Autodesk Inventor part; units mm, degrees
ref_plane "YZ Plane" through (0, 0, 0) normal (1, 0, 0) x (0, 1, 0)
ref_plane "XZ Plane" through (0, 0, 0) normal (0, 1, 0) x (-1, 0, 0)
ref_plane "XY Plane" through (0, 0, 0) normal (0, 0, 1) x (1, 0, 0)
sketch "Sketch1" plane through (0, 0, 0) normal (0, 0, 1) x (1, 0, 0)
  circle A0 centre (0, 0) radius 2.5
  dimension "d0" = 5
extrude "Extrusion1" add sketch "Sketch1" against normal blind 300
sketch "Sketch2" plane through (0, 0, 0) normal (0, 1, 0) x (-1, 0, 0)
  line L0 (1.5, -50) -> (8.5, -50)
  line L1 (8.5, -50) -> (8.5, -100)
  line L2 (8.5, -100) -> (1.5, -100)
  line L3 (1.5, -100) -> (1.5, -50)
  line L4 (1.5, -250) -> (8.5, -250)
  line L5 (8.5, -250) -> (8.5, -200)
  line L6 (8.5, -200) -> (1.5, -200)
  line L7 (1.5, -200) -> (1.5, -250)
  point P0 (0, 0)
  dimension "d3" = 7
  dimension "d4" = 50
  dimension "d5" = 7
  dimension "d6" = 50
  dimension "d7" = 0
  dimension "d8" = 150
  dimension "d9" = 8.5
  dimension "d10" = 50
extrude "Extrusion2" add sketch "Sketch2" along normal mid plane 4
mirror "Mirror1" about plane through (0, 0, 0) normal (1, 0, 0) of "Extrusion2"
sketch "Sketch3" plane through (0, 0, 0) normal (0, 0, 1) x (1, 0, 0)
  circle A0 centre (0, 0) radius 5
  dimension "d13" = 10
extrude "Extrusion3" add sketch "Sketch3" along normal blind 20
properties part number "Rod"
Geometry: final body of the model. Coordinates: model frame, mm. A direction names the side the tool comes from. Round coordinates to 2 decimals unless told otherwise and drop trailing zeros. Write each loop counter-clockwise with the first axis right and the second up, starting at its lowest first coordinate (ties: lowest second). Pieces come first, ordered by that corner, then holes.
Item 1: Section query A-A (z = -221.5). Return loops of the section in (x, y), plus the area to 3 significant figures.
Item 2: Material intervals for L1, parallel to Z at x = -3, y = 1.5; L2, parallel to Z at x = 5.5, y = -1; L3, parallel to Z at x = -0.75, y = 4.75, sorted ascending.
Item 3: Pin query (flat end, axial travel): P1, Ø3, axis at x = 1, z = -199, coming from the -Y side; P2, Ø2, axis at x = -6.5, z = -227.5, coming from the +Y side; P3, Ø2, axis at x = -6, z = -218.5, coming from the -Y side. Return the tip coordinate at first contact, or that it passes through.
Item 4: Set-up query: faces 4 (the face through (-5, -2, -75)), 5 (the face through (-5, 2, -225)), 6 (the face through (-1.08, 4.88, 9.86)). Return all of +Z, -Z, +X, -X, +Y, -Y with unobstructed straight access to the full face (end or side cutting, diameter ignored); none if empty.
Item 5: Mould query, pull axis Z, two halves, no side actions, for faces 1 (the face through (5, 2, -225)), 2 (the face through (2, -2, 0)), 3 (the face through (0, 0, -300)). Classes: +Z half, -Z half, draft (parallel to the pull), parting line (faces both ways), or undercut.
Item 6: Section query B-B (y = 0). Return loops of the section in (x, z).
Completed:
1. outline: (-8.5, -2) - (-1.5, -2) arc R2.5 ccw to (1.5, -2) - (8.5, -2) - (8.5, 2) - (1.5, 2) arc R2.5 ccw to (-1.5, 2) - (-8.5, 2) - close
1. area: 70.0 mm2
2. L1: z = -250 to -200, -100 to -50, 0 to 20
2. L2: z = -250 to -200, -100 to -50
2. L3: z = 0 to 20
3. P1: stops at y = -2.5
3. P2: stops at y = 2
3. P3: stops at y = -2
4. face 4: -Z, -X, -Y
4. face 5: -Z, -X, +Y
4. face 6: +Z
5. face 1: draft
5. face 2: undercut
5. face 3: -Z half
6. outline: (-8.5, -250) - (-2.5, -250) - (-2.5, -300) - (2.5, -300) - (2.5, -250) - (8.5, -250) - (8.5, -200) - (2.5, -200) - (2.5, -100) - (8.5, -100) - (8.5, -50) - (2.5, -50) - (2.5, 0) - (5, 0) - (5, 20) - (-5, 20) - (-5, 0) - (-2.5, 0) - (-2.5, -50) - (-8.5, -50) - (-8.5, -100) - (-2.5, -100) - (-2.5, -200) - (-8.5, -200) - close
